Input: part model. Units: mm. Frame: model coordinates. Face numbers are marked on the shaded views. A direction names the side the tool comes from. Coordinates: 2 decimals unless noted, no trailing zeros. Loops run counter-clockwise (first coordinate to the right, second up) from the corner with the lowest first, then second, coordinate; pieces in that order, holes last. Notation, with made-up numbers: M 38,31 L 79,31 A7 cw 79,36 Z; hole C 26.25,-28 d8. An arc over 180 degrees is marked long. Use a Markdown table: item, result. Add a question column.
1. Section C-C on z = -2.25. Output: boundary loops of the cut face in (x, y).
2. Pin query (flat end, axial travel): pin 1 (2 mm diameter, centred on y = 0.5, z = 1, fed in from -X); pin 2 (1.8 mm diameter, centred on x = 0, z = 0, fed in from +Y); pin 3 (3.5 mm diameter, centred on x = 1, z = 1.5, fed in from -Y). Return the tip coordinate at first contact, or that it passes through.
3. Section D-D on y = 9. Output: boundary loops of the cut face in (x, z), then the cut area to 3 significant figures.
4. Line query: L1, parallel to Z at x = 0, y = 7; L2, parallel to Y at x = -0.5, z = -2; L3, parallel to Y at x = -2.5, z = -0.5. Output: solid intervals per line, ascending. Write a range as [from, to].
5. Draft query along X for the marked faces 1, 2 and 3. Return one class per face: +X half, -X half, draft (parallel to the pull), parting line (faces both ways), or undercut.
6. Set-up query: the marked faces 4, 5 and 6. Return all of +Z, -Z, +X, -X, +Y, -Y with unobstructed straight access to the full face (end or side cutting, diameter ignored); none if empty.
7. Section A-A on y = 2.5. Output: boundary loops of the cut face in (x, z).
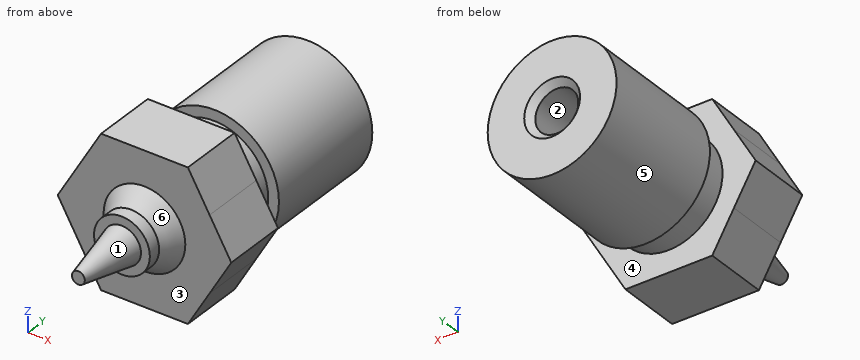
```python
from build123d import *

# Parameters (mm, degrees)
BOSS_EXTRUDE1_DEPTH = 3


with BuildPart() as part:
    # Sketch1 → Revolve1 (revolve)
    with BuildSketch(Plane.XY):
        Polygon((0, 0), (0.5, 0), (1.900415076, 2), (3.5, 2), (3.5, 5), (2.5, 5), (2.5, 6.5), (3, 6.5), (3, 12.5), (0, 12.5), align=None)
    revolve(axis=Axis((0, -1.1291331, 0), (0, -1, 0)))

    # Sketch2 → Cut-Revolve1 (revolve, cut)
    with BuildSketch(Plane.XY):
        Polygon((0, 12.5), (1.3, 12.5), (1, 12.2), (1, 1.985640646), (0.2, 0.6), (0.2, 0), (0, 0), align=None)
    revolve(axis=Axis((0, 0, 0), (0, 1, 0)), mode=Mode.SUBTRACT)

    # Sketch3 → Boss-Extrude1 (add)
    with BuildSketch(Plane.XZ.offset(-2)):
        with BuildLine():
            ThreePointArc((-3.031088921, -1.749999986), (-3.5, 0), (-3.031088921, 1.749999986))
            Line((-3.031088921, 1.749999986), (-4.041451884, 0))
            Line((-4.041451884, 0), (-3.031088921, -1.749999986))
        make_face()
        with BuildLine():
            ThreePointArc((-3.031088921, 1.749999986), (-1.750000007, 3.031088909), (0, 3.5))
            Line((0, 3.5), (-2.020725942, 3.5))
            Line((-2.020725942, 3.5), (-3.031088921, 1.749999986))
        make_face()
        with BuildLine():
            ThreePointArc((0, 3.5), (1.750000007, 3.031088909), (3.031088922, 1.749999985))
            Line((3.031088922, 1.749999985), (2.020725942, 3.5))
            Line((2.020725942, 3.5), (0, 3.5))
        make_face()
        with BuildLine():
            Line((2.020725942, -3.5), (3.031088915, -1.749999996))
            ThreePointArc((3.031088915, -1.749999996), (1.750000009, -3.031088908), (1.6e-08, -3.5))
            Line((1.6e-08, -3.5), (2.020725942, -3.5))
        make_face()
        with BuildLine():
            Line((-2.020725942, -3.5), (1.6e-08, -3.5))
            ThreePointArc((1.6e-08, -3.5), (-1.75, -3.031088913), (-3.031088921, -1.749999986))
            Line((-3.031088921, -1.749999986), (-2.020725942, -3.5))
        make_face()
        with BuildLine():
            Line((3.031088915, -1.749999996), (4.041451884, 0))
            Line((4.041451884, 0), (3.031088922, 1.749999985))
            ThreePointArc((3.031088922, 1.749999985), (3.380740394, 0.90586665), (3.5, 0))
            ThreePointArc((3.5, 0), (3.380740393, -0.905866656), (3.031088915, -1.749999996))
        make_face()
    extrude(amount=-BOSS_EXTRUDE1_DEPTH)

    # Sketch4 → Revolve2 (revolve)
    with BuildSketch(Plane.XY):
        Polygon((0, 0), (0, -2.25), (0.3, -2.25), (0.885114146, 0.55), (1.3, 0.55), (1.3, 2), (1.008290377, 2), (1, 1.985640646), (0.2, 0.6), (0.2, 0), align=None)
    revolve(axis=Axis((0, 2, 0), (0, -1, 0)))


solid = part.part
```
Answers below:
| question | item | result |
|---|---|---|
| 1 | outline | M -2.74,2 L 2.74,2 L 2.74,5 L 1.09,5 L 1.09,6.5 L 1.98,6.5 L 1.98,12.5 L -1.98,12.5 L -1.98,6.5 L -1.09,6.5 L -1.09,5 L -2.74,5 Z |
| 2 | pin 1 | stops at x = -1.37 |
| 2 | pin 2 | stops at y = 1.81 |
| 2 | pin 3 | stops at y = -2.25 |
| 3 | outline | C 0,0 d6; hole C 0,0 d2 |
| 3 | area | 25.1 mm² |
| 4 | L1 | z = [-3, -1], [1, 3] |
| 4 | L2 | y = [2, 12.5] |
| 4 | L3 | y = [2, 5], [6.5, 12.5] |
| 5 | face 1 | parting line |
| 5 | face 2 | undercut |
| 5 | face 3 | draft |
| 6 | face 4 | none |
| 6 | face 5 | +Y |
| 6 | face 6 | -Y |
| 7 | outline | M -4.04,0 L -2.02,-3.5 L 2.02,-3.5 L 4.04,0 L 2.02,3.5 L -2.02,3.5 Z; hole C 0,0 d2 |
